Geometry check sheet. Reference: the model listing, model coordinates, mm. Face numbers are marked on the shaded views. A direction names the side the tool comes from. Round coordinates to 2 decimals unless told otherwise and drop trailing zeros. Order: outer loops, then holes, each group sorted by start corner. A loop starts at its lowest first (then second) coordinate and runs counter-clockwise, first axis right, second up. Notation, with made-up numbers: (67, 51.25) - (106, 51.25) arc R20 cw to (106, 82.25) - close; hole circle Ø2 at (56.5, 9). An arc over 180 degrees is marked (long way). Use a Markdown table: item, result. Add a question column.
(1) Section check D-D on x = 19. Record the boundary of the cut face in (y, z), then the cut area to 3 significant figures.
(2) Mould release check, pull along Z, two halves, no side actions. Record for the marked faces 3, 4 and 5: released by +Z, released by -Z, zero draft, split by the parting line, or undercut.
(3) Access from +Z, -Z, +X, -X, +Y, -Y to the whole of each face (thin tool, end or side, straight path). Record for the marked faces 1 and 2.
(4) Thickness scan on line 1 along Y through (x, z) = (15, -11); line 2 along Y through (x, z) = (20, -19); line 3 along X through (y, z) = (3.2, 0). Record the ranges inside material, lowest first. Write a range as [from, to].
(5) Section check B-B on z = 0. Record the boundary of the cut face in (x, y), then the cut area to 3 significant figures.
(6) Section check A-A on y = 35. Record the boundary of the cut face in (x, z), then the cut area to 3 significant figures.
(7) Gauge pin test, flat ends, axial feed: P1, Ø6, axis at y = 25.5, z = 10.5, coming from the +X side; P2, Ø1.5, axis at x = 19, z = 0, coming from the +Y side; P3, Ø2, axis at x = 17, y = 6, coming from the +Z side; P4, Ø1.5, axis at x = 14.5, z = 4, coming from the -Y side. Record the tip position at first contact, or that the pin passes through.
(8) Section check C-C on x = 0. Record the boundary of the cut face in (y, z).
```python
from build123d import *

# Parameters (mm, degrees)
SKETCH_1_R          = 27.9
EXTRUDE_1_DEPTH     = 45
SKETCH_2_R          = 21.25
CUT_EXTRUDE_1_DEPTH = 30
SKETCH_3_R          = 1.25
CUT_EXTRUDE_2_DEPTH = 6
SKETCH_7_W          = 5
SKETCH_7_H          = 14
CUT_EXTRUDE_3_DEPTH = 45
SKETCH_8_W          = 7
SKETCH_8_H          = 9
CUT_EXTRUDE_4_DEPTH = 90


with BuildPart() as part:
    # Sketch 1 → Extrude 1 (new body)
    with BuildSketch(Plane(origin=(0, 0, 0), x_dir=(1, 0, 0), z_dir=(0, 1, 0))):
        with Locations(Location((0, 0, 0), (0, 0, 90))):
            Circle(SKETCH_1_R)
    extrude(amount=EXTRUDE_1_DEPTH)

    # Sketch 2 → Cut-Extrude 1 (cut)
    with BuildSketch(Plane(origin=(0, 45, 0), x_dir=(1, 0, 0), z_dir=(0, 1, 0))):
        with Locations(Location((0, 0, 0), (0, 0, 270))):
            Circle(SKETCH_2_R)
    extrude(amount=-CUT_EXTRUDE_1_DEPTH, mode=Mode.SUBTRACT)

    # Sketch 3 → Cut-Extrude 2 (cut)
    with BuildSketch(Plane.XZ):
        with Locations(Location((-19, 0, 0), (0, 0, 270))):
            Circle(SKETCH_3_R)
        with Locations(Location((0, 19, 0), (0, 0, 270))):
            Circle(SKETCH_3_R)
        with Locations(Location((19, 0, 0), (0, 0, 270))):
            Circle(SKETCH_3_R)
        with Locations(Location((0, -19, 0), (0, 0, 270))):
            Circle(SKETCH_3_R)
    extrude(amount=-CUT_EXTRUDE_2_DEPTH, mode=Mode.SUBTRACT)

    # Sketch 7 → Cut-Extrude 3 (cut, symmetric)
    with BuildSketch(Plane(origin=(0, 0, 0), x_dir=(0, 1, 0), z_dir=(0.7071067811865438, 0, -0.7071067811865512))):
        with Locations((4, 0)):
            Rectangle(SKETCH_7_W, SKETCH_7_H)
    extrude(amount=CUT_EXTRUDE_3_DEPTH, both=True, mode=Mode.SUBTRACT)

    # Sketch 8 → Cut-Extrude 4 (cut)
    with BuildSketch(Plane(origin=(0, 0, 0), x_dir=(0, 1, 0), z_dir=(0.7071067811865488, 0, 0.7071067811865464))):
        with Locations((5, 0)):
            Rectangle(SKETCH_8_W, SKETCH_8_H)
    extrude(amount=-CUT_EXTRUDE_4_DEPTH, mode=Mode.SUBTRACT)


solid = part.part
```
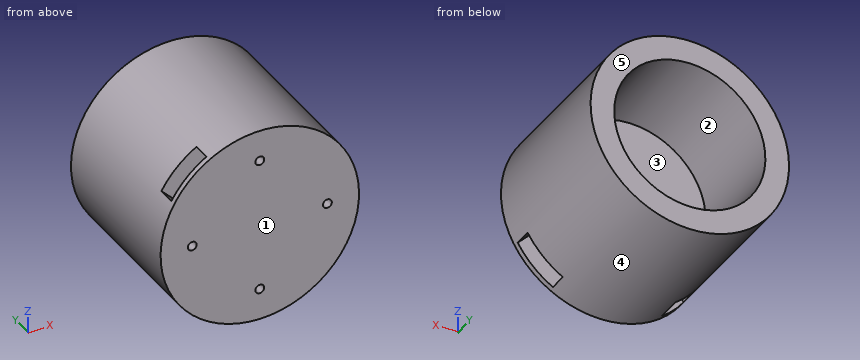
Check sheet entries:
| question | item | result |
|---|---|---|
| 1 | outline | (0, -20.43) - (1.5, -20.43) - (1.5, -9.1) - (6.5, -9.1) - (6.5, -20.43) - (45, -20.43) - (45, -9.52) - (15, -9.52) - (15, 9.52) - (45, 9.52) - (45, 20.43) - (0, 20.43) - (0, 1.25) - (6, 1.25) - (6, -1.25) - (0, -1.25) - close |
| 1 | area | 1,200 mm2 |
| 2 | face 3 | undercut |
| 2 | face 4 | split by the parting line |
| 2 | face 5 | zero draft |
| 3 | face 1 | +Z, -Z, +X, -X, -Y |
| 3 | face 2 | +Y |
| 4 | line 1 | y = [0, 1.5], [6.5, 15] |
| 4 | line 2 | y = [0, 1.5], [6.5, 45] |
| 4 | line 3 | x = [-27.9, -20.25], [-17.75, -9.9], [9.9, 17.75], [20.25, 27.9] |
| 5 | outline | (-27.9, 0) - (-20.25, 0) - (-20.25, 6) - (-17.75, 6) - (-17.75, 0) - (17.75, 0) - (17.75, 6) - (20.25, 6) - (20.25, 0) - (27.9, 0) - (27.9, 45) - (21.25, 45) - (21.25, 15) - (-21.25, 15) - (-21.25, 45) - (-27.9, 45) - close; hole (-9.9, 1.5) - (9.9, 1.5) - (9.9, 6.5) - (0, 6.5) - (0, 8.5) - (-6.36, 8.5) - (-6.36, 6.5) - (-9.9, 6.5) - close |
| 5 | area | 1,090 mm2 |
| 6 | outline | circle Ø55.8 at (0, 0); hole circle Ø42.5 at (0, 0) |
| 6 | area | 1,030 mm2 |
| 7 | P1 | stops at x = 26.87 |
| 7 | P2 | stops at y = 15 |
| 7 | P3 | stops at z = 22.86 |
| 7 | P4 | stops at y = 0 |
| 8 | outline | (0, -27.9) - (45, -27.9) - (45, -21.25) - (15, -21.25) - (15, 21.25) - (45, 21.25) - (45, 27.9) - (0, 27.9) - (0, 20.25) - (6, 20.25) - (6, 17.75) - (0, 17.75) - (0, -17.75) - (6, -17.75) - (6, -20.25) - (0, -20.25) - close; hole (1.5, -9.9) - (6.5, -9.9) - (6.5, -6.36) - (8.5, -6.36) - (8.5, 0) - (6.5, 0) - (6.5, 9.9) - (1.5, 9.9) - close |
